Source: CAD feature listing. Evaluate the final solid. Frame: model axes, mm. A direction names the side the tool comes from. Give positions to 0.01 mm unless a question says otherwise; leave off trailing zeros. Order: outer loops, then holes, each group sorted by start corner. A loop starts at its lowest first (then second) coordinate and runs counter-clockwise, first axis right, second up.
1) Material intervals for line 1 (X direction, y = -0.65, z = 5.35); line 2 (Z direction, x = 5, y = -0.95); line 3 (Y direction, x = 2, z = -1.25), sorted ascending.
2) Access query for faces 1 (the face through (6, 0, 3.6)), 2 (the face through (5, 7.65, -1)), 3 (the face through (5, -1.6, 3)). Directions: +Z, -Z, +X, -X, +Y, -Y. A direction counts if a zero-diameter tool reaches every point of the face in a straight line with its end or side. Return the directions, or none.
3) First-contact query: P1, Ø3, axis at x = 3.5, y = 0.5, coming from the +Z side; P2, Ø6, axis at x = 8, y = 2.5, coming from the -Z side; P3, Ø4, axis at x = 5.5, y = 6.5, coming from the +Z side. Flat tips, straight axial feed; report the tip coordinate or a pass-through.
4) Draft query along Z for faces 4 (the face through (5, 8, -2.5)), 5 (the face through (10, 2, 1)), 6 (the face through (5, 5, 1.6)), 7 (the face through (6.55, -0.81, 6.16)). Return one class per face: released by +Z, released by -Z, zero draft, split by the parting line, or undercut.
5) Section D-D, the plane y = 1. Return loops of the section in (x, z), plus the area to 3 significant figures.
6) Section C-C, the plane x = 0.5. Return loops of the section in (y, z), plus the area to 3 significant figures.
7) Section B-B, the plane z = 5.35. Return loops of the section in (x, y).
8) Section A-A, the plane x = 5. Return loops of the section in (y, z), plus the area to 3 significant figures.
Autodesk Fusion 360 part; units mm, degrees
sketch "Sketch1" plane through (0, 0, 0) normal (0, 1, 0) x (1, 0, 0)
  line L0 (0, 0) -> (10, 0)
  line L1 (10, 0) -> (10, -9.1)
  line L2 (10, -9.1) -> (0, -9.1)
  line L3 (0, -9.1) -> (0, 0)
  line L4 (0, 0) -> (10, 0)
  line L5 (10, 0) -> (10, -1.6)
  line L6 (10, -1.6) -> (0, -1.6)
  line L7 (0, -1.6) -> (0, 0)
  point P0 (5, -5.35)
  dimension "d1" = 1.6
  dimension "d2" = 7.5
  dimension "d3" = 10
  dimension "d10" = 5
  dimension "d11" = 3.75
extrude "Extrude1" add sketch "Sketch1" against normal blind 1.6
extrude "Extrude2" add sketch "Sketch1" along normal blind 9.25 contours L0 L1 L3 L4 L5 L6 L7
sketch "Sketch2" plane through (0, 0, 0) normal (0, 0, -1) x (-1, 0, 0)
  line L0 (-10, 9.25) -> (-10, -1.6)
  line L1 (-10, -1.6) -> (0, -1.6)
  line L2 (0, -1.6) -> (0, 9.25)
  line L3 (0, 9.25) -> (-10, 9.25)
  line L4 (-10, 9.25) -> (0, 9.25)
  line L5 (0, 9.25) -> (0, 7.65)
  line L6 (0, 7.65) -> (-10, 7.65)
  line L7 (-10, 7.65) -> (-10, 9.25)
  dimension "d15" = 1.6
extrude "Extrude3" add sketch "Sketch2" along normal blind 2.5 contours L0 L2 L3 L4 L5 L6 L7
hole "Hole1" at (5, 0, 5.35) direction (0, -1, 0) diameter 3.5 depth 3 tip angle 118
equation "d10 = d3 / 2"
equation "d11 = d2 / 2"
From the geometry:
1. line 1: x = 0 to 3.25, 6.75 to 10
1. line 2: z = 0 to 3.6, 7.1 to 9.1
1. line 3: y = 7.65 to 9.25
2. face 1: +Z, +X, -X, +Y
2. face 2: -Z, +X, -X, -Y
2. face 3: +Z, -Z, +X, -X, -Y
3. P1: stops at z = 9.1
3. P2: stops at z = 0
3. P3: stops at z = 1.6
4. face 4: released by -Z
4. face 5: zero draft
4. face 6: released by +Z
4. face 7: undercut
5. outline: (0, 0) - (10, 0) - (10, 1.6) - (0, 1.6) - close
5. area: 16.0 mm2
6. outline: (-1.6, 0) - (7.65, 0) - (7.65, -2.5) - (9.25, -2.5) - (9.25, 1.6) - (0, 1.6) - (0, 9.1) - (-1.6, 9.1) - close
6. area: 33.4 mm2
7. outline: (0, -1.6) - (3.25, -1.6) - (3.25, 0) - (0, 0) - close; (6.75, -1.6) - (10, -1.6) - (10, 0) - (6.75, 0) - close
8. outline: (-1.6, 0) - (7.65, 0) - (7.65, -2.5) - (9.25, -2.5) - (9.25, 1.6) - (0, 1.6) - (0, 3.6) - (-1.6, 3.6) - close; (-1.6, 7.1) - (0, 7.1) - (0, 9.1) - (-1.6, 9.1) - close
8. area: 27.8 mm2
